Verification items for this drawing (mm, ordinates from the low corner). A direction names the side the tool comes from. Coordinates: 2 decimals unless noted, no trailing zeros. Order: outer loops, then holes, each group sorted by start corner. A loop starts at its lowest first (then second) coordinate and runs counter-clockwise, first axis right, second up. Notation, with made-up numbers: (-21, 53.25) -> (0, 53.25) arc R27 cw to (0, 74.25) -> close; hole circle Ø2 at (-22, 29.5). An arc over 180 degrees is marked (long way). Write each question's results on one line, items separated by ' | '. Start each with the question number.
(1) Set-up check for the marked faces 1 and 2: record each of +Z, -Z, +X, -X, +Y, -Y from which the full face is reachable in a straight line by a thin tool's end or side.
(2) Go/stop test with a flat-tipped pin: pin 1 (1 mm diameter, centred on x = 33.5, y = 22, fed in from +Z). Record where the tip stops, or that it passes through.
(3) Thickness scan on probe 1 along X at (y, z) = (41, 31); probe 2 along Z at (x, y) = (25, 36.5); probe 3 along X at (y, z) = (83, 3). Record the ranges inside material, lowest first. Write a range as [from, to].
(4) Cross-section at A-A on y = 120. Enter the section's corners in (x, z), and give its area (3 significant figures).
(5) Cross-section at C-C on x = 20. Enter the section's corners in (y, z), and give its area (3 significant figures).
(6) Draft check along X on the marked faces 3, 4 and 5. Enter one of: +X half, -X half, draft (parallel to the pull), parting line (faces both ways), or undercut.
(7) Cross-section at B-B on z = 7. Enter the section's corners in (x, y).
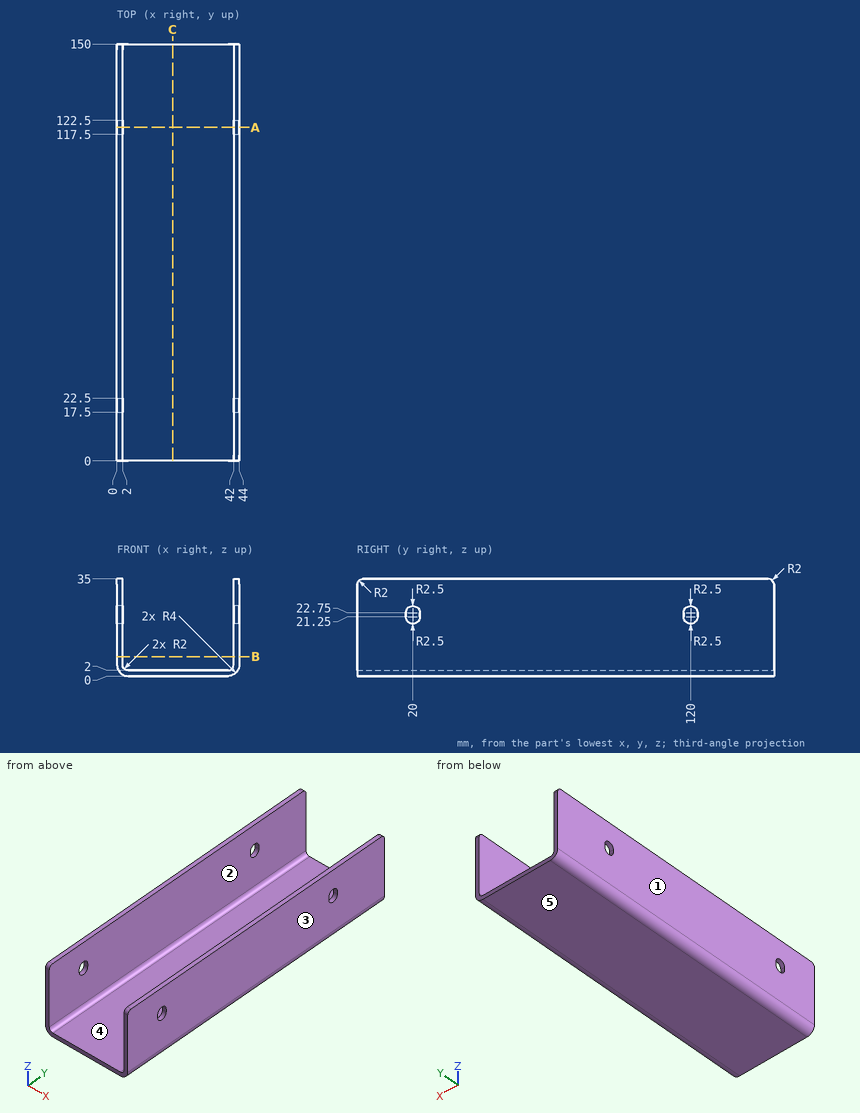
Results are:
1) face 1: +Z, -Z, -X, +Y, -Y | face 2: +Z, +Y, -Y
2) pin 1: stops at z = 2
3) probe 1: x = [0, 2], [42, 44] | probe 2: z = [0, 2] | probe 3: x = [0.13, 2.27], [41.73, 43.87]
4) outline: (0, 4) arc R4 ccw to (4, 0) -> (40, 0) arc R4 ccw to (44, 4) -> (44, 18.75) -> (42, 18.75) -> (42, 4) arc R2 cw to (40, 2) -> (4, 2) arc R2 cw to (2, 4) -> (2, 18.75) -> (0, 18.75) -> close; (0, 25.25) -> (2, 25.25) -> (2, 35) -> (0, 35) -> close; (42, 25.25) -> (44, 25.25) -> (44, 35) -> (42, 35) -> close | area: 189 mm2
5) outline: (0, 0) -> (150, 0) -> (150, 2) -> (0, 2) -> close | area: 300 mm2
6) face 3: +X half | face 4: undercut | face 5: draft
7) outline: (0, 0) -> (2, 0) -> (2, 150) -> (0, 150) -> close; (42, 0) -> (44, 0) -> (44, 150) -> (42, 150) -> close
